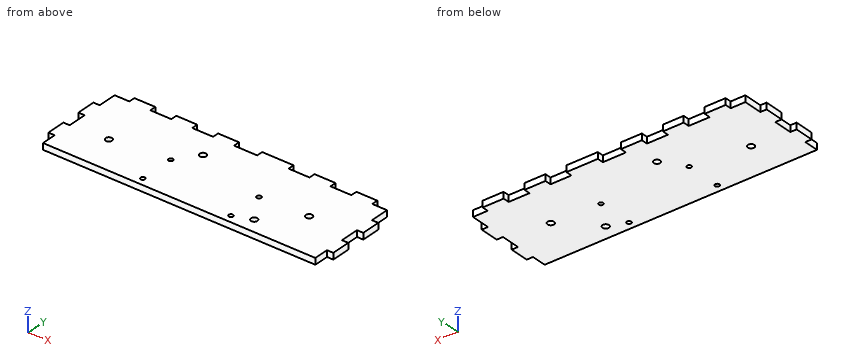
```python
from build123d import *

# Parameters (mm, degrees)
SKETCH1_W           = 136
SKETCH1_H           = 46
BOSS_EXTRUDE1_DEPTH = 3
CUT_EXTRUDE1_REACH  = 5
SKETCH4_W           = 3
SKETCH4_H           = 9
SKETCH4_H_2         = 7
SKETCH4_W_2         = 10
SKETCH4_H_3         = 3
SKETCH4_W_3         = 11
CUT_EXTRUDE2_REACH  = 5
SKETCH5_R           = 1.05
SKETCH5_R_2         = 1.55


with BuildPart() as part:
    # Sketch1 → Boss-Extrude1 (new body)
    with BuildSketch(Plane.XY):
        with Locations((68, 23)):
            Rectangle(SKETCH1_W, SKETCH1_H)
    extrude(amount=BOSS_EXTRUDE1_DEPTH)

    # Sketch4 → Cut-Extrude1 (cut, up to next)
    with BuildSketch(Plane.XY.offset(3), mode=Mode.PRIVATE) as cut_extrude1_sk1:
        Polygon((0, 46), (0, 43), (3, 43), (10, 43), (10, 46), align=None)
    cut_extrude1_tool1 = extrude(cut_extrude1_sk1.sketch, amount=-CUT_EXTRUDE1_REACH, mode=Mode.PRIVATE) & part.part
    add(cut_extrude1_tool1.solids().sort_by_distance((5, 44.5, 3))[0], mode=Mode.SUBTRACT)
    # Sketch4 → Cut-Extrude1 (cut, up to next)
    with BuildSketch(Plane.XY.offset(3), mode=Mode.PRIVATE) as cut_extrude1_sk2:
        with Locations((1.5, 38.5)):
            Rectangle(SKETCH4_W, SKETCH4_H)
    cut_extrude1_tool2 = extrude(cut_extrude1_sk2.sketch, amount=-CUT_EXTRUDE1_REACH, mode=Mode.PRIVATE) & part.part
    add(cut_extrude1_tool2.solids().sort_by_distance((1.5, 38.5, 3))[0], mode=Mode.SUBTRACT)
    # Sketch4 → Cut-Extrude1 (cut, up to next)
    with BuildSketch(Plane.XY.offset(3), mode=Mode.PRIVATE) as cut_extrude1_sk3:
        with Locations((1.5, 20.5)):
            Rectangle(SKETCH4_W, SKETCH4_H)
    cut_extrude1_tool3 = extrude(cut_extrude1_sk3.sketch, amount=-CUT_EXTRUDE1_REACH, mode=Mode.PRIVATE) & part.part
    add(cut_extrude1_tool3.solids().sort_by_distance((1.5, 20.5, 3))[0], mode=Mode.SUBTRACT)
    # Sketch4 → Cut-Extrude1 (cut, up to next)
    with BuildSketch(Plane.XY.offset(3), mode=Mode.PRIVATE) as cut_extrude1_sk4:
        with Locations((1.5, 3.5)):
            Rectangle(SKETCH4_W, SKETCH4_H_2)
    cut_extrude1_tool4 = extrude(cut_extrude1_sk4.sketch, amount=-CUT_EXTRUDE1_REACH, mode=Mode.PRIVATE) & part.part
    add(cut_extrude1_tool4.solids().sort_by_distance((1.5, 3.5, 3))[0], mode=Mode.SUBTRACT)
    # Sketch4 → Cut-Extrude1 (cut, up to next)
    with BuildSketch(Plane.XY.offset(3), mode=Mode.PRIVATE) as cut_extrude1_sk5:
        with Locations((25, 44.5)):
            Rectangle(SKETCH4_W_2, SKETCH4_H_3)
    cut_extrude1_tool5 = extrude(cut_extrude1_sk5.sketch, amount=-CUT_EXTRUDE1_REACH, mode=Mode.PRIVATE) & part.part
    add(cut_extrude1_tool5.solids().sort_by_distance((25, 44.5, 3))[0], mode=Mode.SUBTRACT)
    # Sketch4 → Cut-Extrude1 (cut, up to next)
    with BuildSketch(Plane.XY.offset(3), mode=Mode.PRIVATE) as cut_extrude1_sk6:
        with Locations((45, 44.5)):
            Rectangle(SKETCH4_W_2, SKETCH4_H_3)
    cut_extrude1_tool6 = extrude(cut_extrude1_sk6.sketch, amount=-CUT_EXTRUDE1_REACH, mode=Mode.PRIVATE) & part.part
    add(cut_extrude1_tool6.solids().sort_by_distance((45, 44.5, 3))[0], mode=Mode.SUBTRACT)
    # Sketch4 → Cut-Extrude1 (cut, up to next)
    with BuildSketch(Plane.XY.offset(3), mode=Mode.PRIVATE) as cut_extrude1_sk7:
        with Locations((65.5, 44.5)):
            Rectangle(SKETCH4_W_3, SKETCH4_H_3)
    cut_extrude1_tool7 = extrude(cut_extrude1_sk7.sketch, amount=-CUT_EXTRUDE1_REACH, mode=Mode.PRIVATE) & part.part
    add(cut_extrude1_tool7.solids().sort_by_distance((65.5, 44.5, 3))[0], mode=Mode.SUBTRACT)
    # Sketch4 → Cut-Extrude1 (cut, up to next)
    with BuildSketch(Plane.XY.offset(3), mode=Mode.PRIVATE) as cut_extrude1_sk8:
        with Locations((91, 44.5)):
            Rectangle(SKETCH4_W_2, SKETCH4_H_3)
    cut_extrude1_tool8 = extrude(cut_extrude1_sk8.sketch, amount=-CUT_EXTRUDE1_REACH, mode=Mode.PRIVATE) & part.part
    add(cut_extrude1_tool8.solids().sort_by_distance((91, 44.5, 3))[0], mode=Mode.SUBTRACT)
    # Sketch4 → Cut-Extrude1 (cut, up to next)
    with BuildSketch(Plane.XY.offset(3), mode=Mode.PRIVATE) as cut_extrude1_sk9:
        with Locations((111, 44.5)):
            Rectangle(SKETCH4_W_2, SKETCH4_H_3)
    cut_extrude1_tool9 = extrude(cut_extrude1_sk9.sketch, amount=-CUT_EXTRUDE1_REACH, mode=Mode.PRIVATE) & part.part
    add(cut_extrude1_tool9.solids().sort_by_distance((111, 44.5, 3))[0], mode=Mode.SUBTRACT)
    # Sketch4 → Cut-Extrude1 (cut, up to next)
    with BuildSketch(Plane.XY.offset(3), mode=Mode.PRIVATE) as cut_extrude1_sk10:
        Polygon((133, 43), (136, 43), (136, 46), (126, 46), (126, 43), align=None)
    cut_extrude1_tool10 = extrude(cut_extrude1_sk10.sketch, amount=-CUT_EXTRUDE1_REACH, mode=Mode.PRIVATE) & part.part
    add(cut_extrude1_tool10.solids().sort_by_distance((131, 44.5, 3))[0], mode=Mode.SUBTRACT)
    # Sketch4 → Cut-Extrude1 (cut, up to next)
    with BuildSketch(Plane.XY.offset(3), mode=Mode.PRIVATE) as cut_extrude1_sk11:
        with Locations((134.5, 38.5)):
            Rectangle(SKETCH4_W, SKETCH4_H)
    cut_extrude1_tool11 = extrude(cut_extrude1_sk11.sketch, amount=-CUT_EXTRUDE1_REACH, mode=Mode.PRIVATE) & part.part
    add(cut_extrude1_tool11.solids().sort_by_distance((134.5, 38.5, 3))[0], mode=Mode.SUBTRACT)
    # Sketch4 → Cut-Extrude1 (cut, up to next)
    with BuildSketch(Plane.XY.offset(3), mode=Mode.PRIVATE) as cut_extrude1_sk12:
        with Locations((134.5, 20.5)):
            Rectangle(SKETCH4_W, SKETCH4_H)
    cut_extrude1_tool12 = extrude(cut_extrude1_sk12.sketch, amount=-CUT_EXTRUDE1_REACH, mode=Mode.PRIVATE) & part.part
    add(cut_extrude1_tool12.solids().sort_by_distance((134.5, 20.5, 3))[0], mode=Mode.SUBTRACT)
    # Sketch4 → Cut-Extrude1 (cut, up to next)
    with BuildSketch(Plane.XY.offset(3), mode=Mode.PRIVATE) as cut_extrude1_sk13:
        with Locations((134.5, 3.5)):
            Rectangle(SKETCH4_W, SKETCH4_H_2)
    cut_extrude1_tool13 = extrude(cut_extrude1_sk13.sketch, amount=-CUT_EXTRUDE1_REACH, mode=Mode.PRIVATE) & part.part
    add(cut_extrude1_tool13.solids().sort_by_distance((134.5, 3.5, 3))[0], mode=Mode.SUBTRACT)

    # Sketch5 → Cut-Extrude2 (cut, up to next)
    with BuildSketch(Plane(origin=(0, 0, 0), x_dir=(-1, 0, 0), z_dir=(0, 0, -1)), mode=Mode.PRIVATE) as cut_extrude2_sk1:
        with Locations((-89.8, 20.5)):
            Circle(SKETCH5_R)
    cut_extrude2_tool1 = extrude(cut_extrude2_sk1.sketch, amount=-CUT_EXTRUDE2_REACH, mode=Mode.PRIVATE) & part.part
    add(cut_extrude2_tool1.solids().sort_by_distance((89.8, 20.5, 0))[0], mode=Mode.SUBTRACT)
    # Sketch5 → Cut-Extrude2 (cut, up to next)
    with BuildSketch(Plane(origin=(0, 0, 0), x_dir=(-1, 0, 0), z_dir=(0, 0, -1)), mode=Mode.PRIVATE) as cut_extrude2_sk2:
        with Locations((-89.8, 3.7)):
            Circle(SKETCH5_R)
    cut_extrude2_tool2 = extrude(cut_extrude2_sk2.sketch, amount=-CUT_EXTRUDE2_REACH, mode=Mode.PRIVATE) & part.part
    add(cut_extrude2_tool2.solids().sort_by_distance((89.8, 3.7, 0))[0], mode=Mode.SUBTRACT)
    # Sketch5 → Cut-Extrude2 (cut, up to next)
    with BuildSketch(Plane(origin=(0, 0, 0), x_dir=(-1, 0, 0), z_dir=(0, 0, -1)), mode=Mode.PRIVATE) as cut_extrude2_sk3:
        with Locations((-47.7, 20.5)):
            Circle(SKETCH5_R)
    cut_extrude2_tool3 = extrude(cut_extrude2_sk3.sketch, amount=-CUT_EXTRUDE2_REACH, mode=Mode.PRIVATE) & part.part
    add(cut_extrude2_tool3.solids().sort_by_distance((47.7, 20.5, 0))[0], mode=Mode.SUBTRACT)
    # Sketch5 → Cut-Extrude2 (cut, up to next)
    with BuildSketch(Plane(origin=(0, 0, 0), x_dir=(-1, 0, 0), z_dir=(0, 0, -1)), mode=Mode.PRIVATE) as cut_extrude2_sk4:
        with Locations((-47.7, 3.7)):
            Circle(SKETCH5_R)
    cut_extrude2_tool4 = extrude(cut_extrude2_sk4.sketch, amount=-CUT_EXTRUDE2_REACH, mode=Mode.PRIVATE) & part.part
    add(cut_extrude2_tool4.solids().sort_by_distance((47.7, 3.7, 0))[0], mode=Mode.SUBTRACT)
    # Sketch5 → Cut-Extrude2 (cut, up to next)
    with BuildSketch(Plane(origin=(0, 0, 0), x_dir=(-1, 0, 0), z_dir=(0, 0, -1)), mode=Mode.PRIVATE) as cut_extrude2_sk5:
        with Locations((-20.677552724, 17.314204089)):
            Circle(SKETCH5_R_2)
    cut_extrude2_tool5 = extrude(cut_extrude2_sk5.sketch, amount=-CUT_EXTRUDE2_REACH, mode=Mode.PRIVATE) & part.part
    add(cut_extrude2_tool5.solids().sort_by_distance((20.677553, 17.314204, 0))[0], mode=Mode.SUBTRACT)
    # Sketch5 → Cut-Extrude2 (cut, up to next)
    with BuildSketch(Plane(origin=(0, 0, 0), x_dir=(-1, 0, 0), z_dir=(0, 0, -1)), mode=Mode.PRIVATE) as cut_extrude2_sk6:
        with Locations((-55, 30.651276125)):
            Circle(SKETCH5_R_2)
    cut_extrude2_tool6 = extrude(cut_extrude2_sk6.sketch, amount=-CUT_EXTRUDE2_REACH, mode=Mode.PRIVATE) & part.part
    add(cut_extrude2_tool6.solids().sort_by_distance((55, 30.651276, 0))[0], mode=Mode.SUBTRACT)
    # Sketch5 → Cut-Extrude2 (cut, up to next)
    with BuildSketch(Plane(origin=(0, 0, 0), x_dir=(-1, 0, 0), z_dir=(0, 0, -1)), mode=Mode.PRIVATE) as cut_extrude2_sk7:
        with Locations((-112.926148706, 21.541179951)):
            Circle(SKETCH5_R_2)
    cut_extrude2_tool7 = extrude(cut_extrude2_sk7.sketch, amount=-CUT_EXTRUDE2_REACH, mode=Mode.PRIVATE) & part.part
    add(cut_extrude2_tool7.solids().sort_by_distance((112.926149, 21.54118, 0))[0], mode=Mode.SUBTRACT)
    # Sketch5 → Cut-Extrude2 (cut, up to next)
    with BuildSketch(Plane(origin=(0, 0, 0), x_dir=(-1, 0, 0), z_dir=(0, 0, -1)), mode=Mode.PRIVATE) as cut_extrude2_sk8:
        with Locations((-98.323238206, 6.929404951)):
            Circle(SKETCH5_R_2)
    cut_extrude2_tool8 = extrude(cut_extrude2_sk8.sketch, amount=-CUT_EXTRUDE2_REACH, mode=Mode.PRIVATE) & part.part
    add(cut_extrude2_tool8.solids().sort_by_distance((98.323238, 6.929405, 0))[0], mode=Mode.SUBTRACT)


solid = part.part
```
Read the model definition and answer for the solid it produces. Units are mm, in the model's axes. Give positions to 0.01 mm unless a question says otherwise; leave off trailing zeros. Write each loop counter-clockwise with the first axis right and the second up, starting at its lowest first coordinate (ties: lowest second). Pieces come first, ordered by that corner, then holes. Notation, with made-up numbers: (-30.5, -30.5) -> (5.5, -30.5) arc R25 ccw to (5.5, 5.5) -> close; hole circle Ø2 at (87.25, -22.5). An arc over 180 degrees is marked (long way). Answer in a Markdown table with one row per item.
1) Section D-D on z = 1.6 is taken. Count the separate pieces of the cut face and the enclosed holes in it, plus the area to 3 significant figures.
Results list:
| item | result |
|---|---|
| separate pieces | 1 |
| enclosed holes | 8 |
| area | 5,850 mm^2 |
2) Section A-A on x = 55 is taken. Give the vertices of the cut face in (y, z).
Results list:
| item | result |
|---|---|
| outline | (0, 0) -> (29.1, 0) -> (29.1, 3) -> (0, 3) -> close; (32.2, 0) -> (46, 0) -> (46, 3) -> (32.2, 3) -> close |
3) Section B-B on y = 38.5 is taken. Give the vertices of the cut face in (x, z).
Results list:
| item | result |
|---|---|
| outline | (3, 0) -> (133, 0) -> (133, 3) -> (3, 3) -> close |
4) Straight lines are drawn through the part: line 1 (X direction, y = 43.5, z = 1.1); line 2 (Y direction, x = 89.8, z = 1.2); line 3 (Y direction, x = 63.5, z = 0.8). For each, find the intervals that lie inside material, in ascending order. Write a range as [from, to].
Results list:
| item | result |
|---|---|
| line 1 | [10, 20], [30, 40], [50, 60], [71, 86], [96, 106], [116, 126] |
| line 2 | [0, 2.65], [4.75, 19.45], [21.55, 43] |
| line 3 | [0, 43] |
5) Section C-C on x = 127.5 is taken. Give the vertices of the cut face in (y, z).
Results list:
| item | result |
|---|---|
| outline | (0, 0) -> (43, 0) -> (43, 3) -> (0, 3) -> close |
6) Each of these flat-tipped pins is pushed along its axis until it touches: pin 1 Ø0.9 at (y, z) = (44, 1) entering from -X; pin 2 Ø0.9 at (y, z) = (45, 1) entering from +X; pin 3 Ø1.5 at (x, z) = (134.5, 1.5) entering from -Y. Where does it stop, or does it pass through?
Results list:
| item | result |
|---|---|
| pin 1 | x = 10 |
| pin 2 | x = 126 |
| pin 3 | y = 7 |
